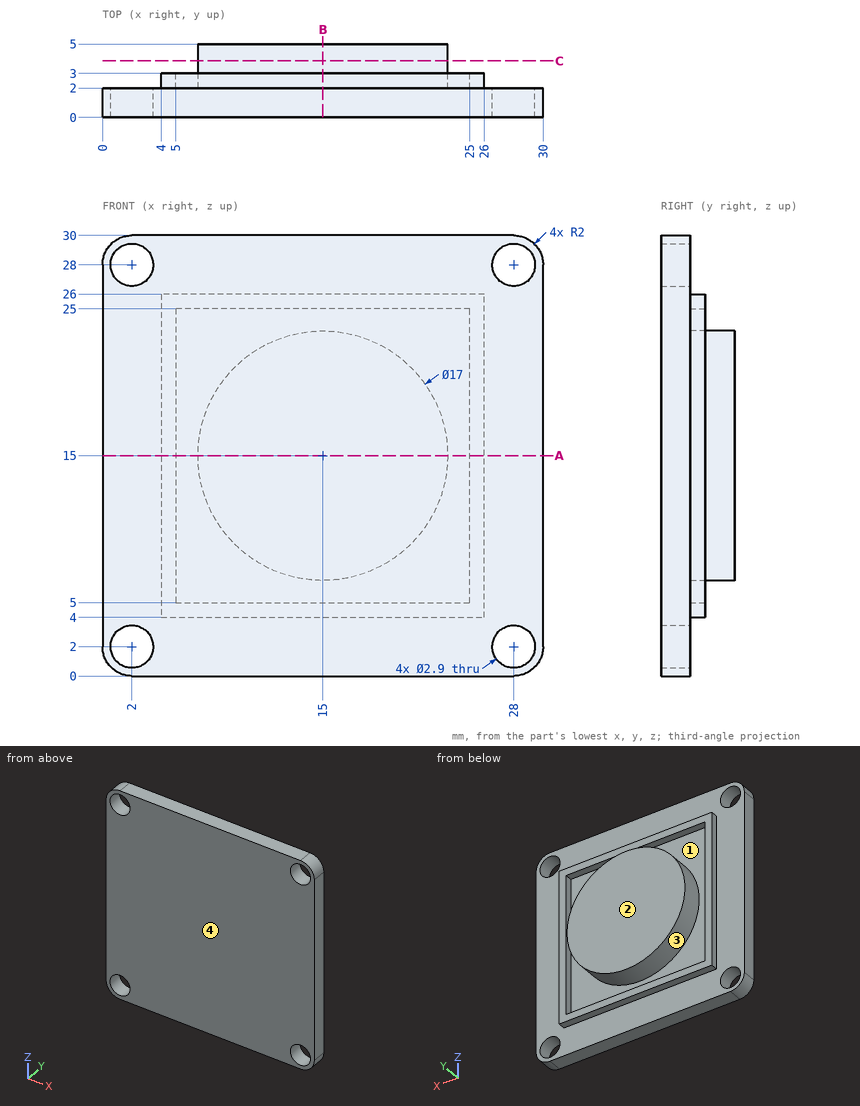
Study the drawing (mm; zero at the part's minimum x, y, z) and answer. A direction names the side the tool comes from. Round coordinates to 2 decimals unless told otherwise and drop trailing zeros. Loops run counter-clockwise (first coordinate to the right, second up) from the corner with the lowest first, then second, coordinate; pieces in that order, holes last.
Q1. Section C-C, the plane y = 3.85 is taken. Determine the outline of the cut face in (x, z).
Q2. Which of the six approach directions +Z, -Z, +X, -X, +Y, -Y give full straight-line access (tool end or side, diameter ignored) to the marked faces 1 and 2?
Q3. Find the intervals of material crossed by line 1 (X direction, y = 1.4, z = 2); line 2 (X direction, y = 2.4, z = 6.25), in increasing order.
Q4. For a pull along Z with two mould halves and no side action, classify the marked faces 3 and 4 as released by +Z, released by -Z, zero draft, split by the parting line, or undercut.
Q5. Section A-A, the plane z = 15 is taken. Determine the outline of the cut face in (x, y).
Q6. Section B-B, the plane x = 15 is taken. Determine the outline of the cut face in (y, z).
Q7. Given pin 1 Ø0.5 at (y, z) = (2.5, 20) entering from -X; pin 2 Ø3.5 at (x, z) = (2, 2) entering from +Y, each flat-ended and moving along its own axis, determine where each tip first touches the part or whether it passes through.
Completed:
1. outline: circle Ø17 at (15, 15)
2. face 1: +Y
2. face 2: +Z, -Z, +X, -X, +Y
3. line 1: x = 0 to 0.55, 3.45 to 26.55, 29.45 to 30
3. line 2: x = 4 to 5, 25 to 26
4. face 3: undercut
4. face 4: zero draft
5. outline: (0, 0) - (30, 0) - (30, 2) - (26, 2) - (26, 3) - (25, 3) - (25, 2) - (23.5, 2) - (23.5, 5) - (6.5, 5) - (6.5, 2) - (5, 2) - (5, 3) - (4, 3) - (4, 2) - (0, 2) - close
6. outline: (0, 0) - (2, 0) - (2, 4) - (3, 4) - (3, 5) - (2, 5) - (2, 6.5) - (5, 6.5) - (5, 23.5) - (2, 23.5) - (2, 25) - (3, 25) - (3, 26) - (2, 26) - (2, 30) - (0, 30) - close
7. pin 1: stops at x = 4
7. pin 2: stops at y = 2
